Job drawing, mm, ordinate dimensions from the low corner. One solid piece. Give positions to 0.01 mm unless a question says otherwise; leave off trailing zeros. Order: outer loops, then holes, each group sorted by start corner. A loop starts at its lowest first (then second) coordinate and runs counter-clockwise, first axis right, second up. Notation, with made-up numbers: M 59,-26.5 L 68,-26.5 A18 ccw 68,7.5 Z; hole C 8,-28 d11. An arc over 180 degrees is marked long. Use CSV: the item, a comma, the result in double quotes. Start each with the question number.
Item 1: Band-saw the part on C-C on z = 2.85. Write the cut outline in (x, y), plus the area to 3 significant figures.
Item 2: Pin check, flat tip, straight feed: P1, Ø11, axis at x = 312, y = 482, coming from the -Z side. Stop position of the tip, or through.
Item 3: Wall check: line 1 along Y through (x, z) = (312, 2.1); line 2 along X through (y, z) = (482, 1.4); line 3 along Y through (x, z) = (192, 3.1). Give the ranges that are in metal, low to high.
Item 4: Band-saw the part on A-A on y = 302. Write the cut outline in (x, z), plus the area to 3 significant figures.
Item 5: Band-saw the part on B-B on x = 192. Write the cut outline in (y, z).
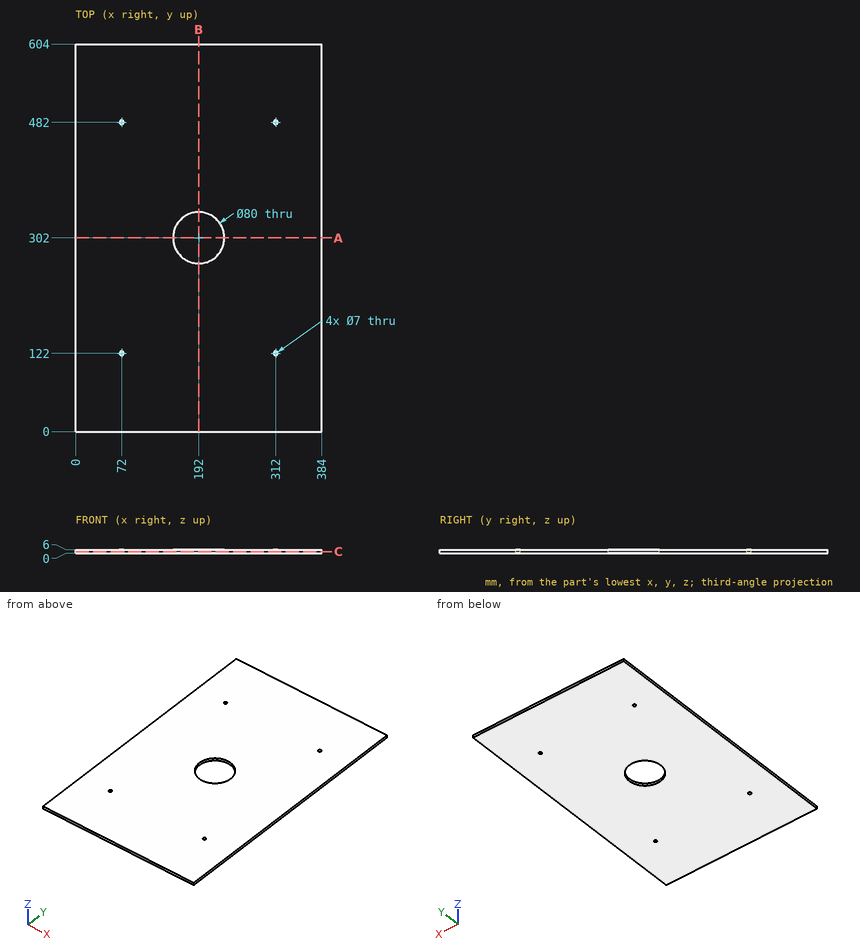
Model answer:
1,outline,"M 0,0 L 384,0 L 384,604 L 0,604 Z; hole C 72,122 d7; hole C 72,482 d7; hole C 192,302 d80; hole C 312,122 d7; hole C 312,482 d7"
1,area,"227,000 mm^2"
2,P1,"stops at z = 0"
3,line 1,"y = 0 to 118.5, 125.5 to 478.5, 485.5 to 604"
3,line 2,"x = 0 to 68.5, 75.5 to 308.5, 315.5 to 384"
3,line 3,"y = 0 to 262, 342 to 604"
4,outline,"M 0,0 L 152,0 L 152,6 L 0,6 Z; M 232,0 L 384,0 L 384,6 L 232,6 Z"
4,area,"1,820 mm^2"
5,outline,"M 0,0 L 262,0 L 262,6 L 0,6 Z; M 342,0 L 604,0 L 604,6 L 342,6 Z"
